The model under review builds one solid part; all positions refer to its coordinate system, in mm. Face numbers are marked on the shaded views. Coordinates: 2 decimals unless noted, no trailing zeros. Loops run counter-clockwise (first coordinate to the right, second up) from the corner with the lowest first, then second, coordinate; pieces in that order, holes last. Notation, with made-up numbers: M 86.25,55.25 L 106.25,55.25 A16 ccw 106.25,65.25 Z; hole C 12,41 d6. An arc over 180 degrees is marked long. Use one line per item in the form item = value.
Autodesk Inventor part; units mm, degrees
ref_plane "作業平面1" through (0, -0.65, 0) normal (0, 1, 0) x (1, 0, 0)
ref_plane "YZ Plane" through (0, 0, 0) normal (1, 0, 0) x (0, 1, 0)
ref_plane "XZ Plane" through (0, 0, 0) normal (0, 1, 0) x (-1, 0, 0)
sketch "スケッチ1" plane through (0, 0, 0) normal (0, 1, 0) x (-1, 0, 0)
  circle A0 centre (0, 0) radius 8.9
  line L0 (0, -8.9) -> (63.2748, -8.9)
  line L1 (63.2748, -8.9) -> (63.2748, 8.9)
  line L2 (63.2748, 8.9) -> (0, 8.9)
  line L3 (0, 8.9) -> (0, -8.9)
  circle A1 centre (0, 0) radius 8.4
  line L4 (0, -8.4) -> (63.2748, -8.4)
  line L5 (63.2748, -8.4) -> (63.2748, 8.4)
  line L6 (63.2748, 8.4) -> (0, 8.4)
  line L7 (0, 8.4) -> (0, -8.4)
  point P0 (0, 8.4)
  point P1 (0, 8.9)
  dimension "d0" = 17.8
  dimension "d1" = 16.8
extrude "押し出し1" add sketch "スケッチ1" along normal blind 0.85 contours L3 A1 A0 | L2 L1 L6 A0 | A0 L6 L3 | L3 L4 A0 | A0 L4 L1 L0
sketch "スケッチ2" plane through (0, 0.85, 0) normal (0, 1, 0) x (1, 0, 0)
  circle A0 centre (0, 0) radius 12
  line L0 (0, 12) -> (-63.2748, 12)
  line L1 (-63.2748, 12) -> (-63.2748, -12)
  line L2 (-63.2748, -12) -> (0, -12)
  line L3 (0, -12) -> (0, 12)
  line L4 (-63.2748, 8.9) -> (-63.2748, 8.4)
  line L5 (-63.2748, 8.4) -> (0, 8.4)
  line L6 (0, -8.4) -> (-63.2748, -8.4)
  arc A1 (0, -8.4) -> (0, 8.4) centre (0, 0) ccw
  point P0 (0, -12)
  dimension "d4" = 24
extrude "押し出し2" add sketch "スケッチ2" along normal blind 1 contours A0 L3 A1 | L3 L5 A0 | A0 L5 L1 L0 | L2 L1 L6 A0 | A0 L6 L3
mirror "ミラー1" about plane through (-27.1874, 0, 0) normal (0, -1, 0)
sketch "スケッチ3" plane through (0, 1.85, 0) normal (0, 1, 0) x (1, 0, 0)
  line L0 (-14.7409, 17.0236) -> (-35.8476, -19.5343)
  line L1 (0, -8.4) -> (-63.2748, -8.4)
  line L2 (-63.2748, -8.4) -> (-63.2748, -12)
  line L3 (-63.2748, -12) -> (0, -12)
  arc A0 (0, -12) -> (0, 12) centre (0, 0) ccw
  line L4 (0, 12) -> (-63.2748, 12)
  line L5 (-63.2748, 12) -> (-63.2748, 8.4)
  line L6 (-63.2748, 8.4) -> (0, 8.4)
  arc A1 (0, -8.4) -> (0, 8.4) centre (0, 0) ccw
  point P0 (-31.4977, -12)
  point P1 (-29.4192, -8.4)
  point P2 (-19.7197, 8.4)
  point P3 (-17.6412, 12)
extrude "押し出し3" cut sketch "スケッチ3" against normal through all contours L0 L6 L5 L4 | L0 L3 L2 L1
ref_plane "作業平面1" through (0, -0.65, 0) normal (0, 1, 0) x (1, 0, 0)
sketch "スケッチ4" plane through (0, -0.65, 0) normal (0, 1, 0) x (1, 0, 0)
  line L0 (-19.7197, 8.4) -> (0, 8.4)
  arc A0 (0, -8.4) -> (0, 8.4) centre (0, 0) ccw
  line L1 (0, -8.4) -> (-29.4192, -8.4)
  line L2 (-19.7197, 8.4) -> (-29.4192, -8.4)
  circle A1 centre (0, 0) radius 1.6
  dimension "d10" = 3.2
extrude "押し出し4" add sketch "スケッチ4" along normal up to surface (2.5 mm away)
fillet "フィレット1" radius 1 3 edges at (-9.8599, -0.65, -8.4) (8.4, -0.65, 0) (-14.7096, -0.65, 8.4)
sketch "スケッチ5" plane through (0, 1.85, 0) normal (0, 1, 0) x (1, 0, 0)
  circle A0 centre (-27.8315, -17.35) radius 1.6
  circle A1 centre (-8.7282, 17.4379) radius 1.6
  line L0 (0, 12) -> (-17.6412, 12)
  line L1 (-17.6412, 12) -> (-10.5885, 24.2158)
  line L2 (-10.5885, 24.2158) -> (0, 24.2158)
  line L3 (-39.933, -26.6105) -> (-10.6554, 24.0998)
  line L4 (0, 12) -> (-17.6412, 12)
  circle A2 centre (0, 0) radius 24.2158
  arc A3 (0, -12) -> (0, 12) centre (0, 0) ccw
  line L5 (11.4695, 3.5285) -> (5.2849, 23.6321)
  circle A4 centre (1.9592, 17.4379) radius 1.6
  line L6 (-39.933, -26.6105) -> (-10.6554, 24.0998)
  circle A5 centre (-31.9338, -24.4553) radius 1.6
  circle A6 centre (-36, -34.6362) radius 1.6
  circle A7 centre (-27.8315, -17.35) radius 1.6
  line L7 (-39.933, -26.6105) -> (-10.6554, 24.0998)
  line L8 (-40, -50) -> (-40, -26.8605)
  line L9 (-38, -50.5) -> (-39.5, -50.5)
  line L10 (-31, -42) -> (-31, -32.0566)
  line L11 (-30.933, -31.8066) -> (-18.1986, -9.75)
  line L12 (-37.5, -50) -> (-37.5, -43)
  line L13 (-37, -42.5) -> (-31.5, -42.5)
  circle A8 centre (-31.9338, -24.4553) radius 5.85
  arc A9 (19.2639, -16.134) -> (19.9469, -15.951) centre (19.5139, -15.701) ccw
  line L14 (29.8557, 1.2115) -> (19.9469, -15.951)
  arc A10 (29.8557, 1.2115) -> (29.8557, 1.7115) centre (29.4226, 1.4615) ccw
  line L15 (10.25, 35.6695) -> (29.8557, 1.7115)
  arc A11 (10.25, 35.6695) -> (9.567, 35.8525) centre (9.817, 35.4195) ccw
  line L16 (-10.4724, 24.2828) -> (9.567, 35.8525)
  arc A12 (-10.4724, 24.2828) -> (-10.6554, 24.0998) centre (-10.2224, 23.8498) ccw
  arc A13 (-39.933, -26.6105) -> (-40, -26.8605) centre (-39.5, -26.8605) ccw
  arc A14 (-40, -50) -> (-39.5, -50.5) centre (-39.5, -50) ccw
  arc A15 (-38, -50.5) -> (-37.5, -50) centre (-38, -50) ccw
  arc A16 (-37, -42.5) -> (-37.5, -43) centre (-37, -43) ccw
  arc A17 (-31.5, -42.5) -> (-31, -42) centre (-31.5, -42) ccw
  arc A18 (-30.933, -31.8066) -> (-31, -32.0566) centre (-30.5, -32.0566) ccw
  arc A19 (-17.7656, -9.5) -> (-18.1986, -9.75) centre (-17.7656, -10) ccw
  line L17 (-17.7656, -9.5) -> (7.6395, -9.5)
  arc A20 (7.8895, -9.567) -> (7.6395, -9.5) centre (7.6395, -10) ccw
  line L18 (7.8895, -9.567) -> (19.2639, -16.134)
  circle A21 centre (1.9592, 17.4379) radius 1.6
  circle A22 centre (24.5152, 1.2615) radius 1.6
  circle A23 centre (5.1388, 27.5224) radius 1.6
  circle A24 centre (13.1994, 17.561) radius 1.6
  circle A25 centre (20.4199, -5.8317) radius 1.6
  circle A26 centre (-8.7282, 17.4379) radius 1.6
  circle A27 centre (0, 0) radius 1.5
  point P0 (0, 24.2158)
  point P1 (-20.2427, -13.2905)
  point P2 (-12.6465, 20.6512)
  point P3 (-37, -21.5303)
  point P4 (-29.8432, -29.9191)
  point P5 (-26.1568, -23.5339)
  dimension "d14" = 15
  dimension "d15" = 3.2
  dimension "d16" = 5
extrude "押し出し5" add sketch "スケッチ5" against normal blind 1 contours A1 | A3 L17 A19 L11 A2 L3 L0 | L0 L1 A2 L5 A3 | L5 A2 A22 L18 A20 L17 A3 | L1 A12 L2 A2 | A2 L11 A8 L3 | A2 L2 A12 L16 A11 L15 A10 L14 A9 L18 A22 | L1 L2 A12 | A8 L11 A18 L10 A17 L13 A16 L12 A15 L9 A14 L8 A13 L3 | A8 L11 | A22 A2 | A2 A22 | A8 L11 | A4 | A6 | A23 | A24 | A25 | A27
sketch "スケッチ6" plane through (0, 1.85, 0) normal (0, 1, 0) x (1, 0, 0)
  line L0 (-19.4977, -12) -> (0, -12)
  line L1 (-19.4977, -12) -> (-17.7656, -9)
  line L2 (-17.7656, -9) -> (7.9373, -9)
  arc A0 (0, -12) -> (0, 12) centre (0, 0) ccw
  line L3 (-29.8432, -29.9191) -> (-19.4977, -12)
  point P0 (-25.741, -22.8137)
  point P1 (-20.2427, -13.2905)
  point P2 (-31, -31.9226)
  dimension "d19" = 3
extrude "押し出し6" cut sketch "スケッチ6" against normal through all
sketch "スケッチ7" plane through (0, -1.85, 0) normal (0, -1, 0) x (1, 0, 0)
  line L0 (-19.3733, -9) -> (0, -9)
  line L1 (-17.7656, 9) -> (-19.4977, 12)
  line L2 (-31.4977, 12) -> (-19.4977, 12)
  line L3 (-31.4977, 12) -> (-29.4192, 8.4)
  line L4 (0, 8.4) -> (-29.4192, 8.4)
  arc A0 (0, -8.4) -> (0, 8.4) centre (0, 0) ccw
  line L5 (-19.7197, -8.4) -> (0, -8.4)
  line L6 (-19.7197, -8.4) -> (-17.6412, -12)
  line L7 (0, -12) -> (-17.6412, -12)
  arc A1 (0, -12) -> (7.9373, 9) centre (0, 0) ccw
  line L8 (7.9373, 9) -> (-17.7656, 9)
  circle A2 centre (0, 0) radius 1.6
  line L9 (0, -7.4) -> (-20.2971, -7.4)
  arc A3 (0, -7.4) -> (0, 7.4) centre (0, 0) ccw
  line L10 (-28.8418, 7.4) -> (0, 7.4)
  line L11 (-20.2971, -7.4) -> (-28.8418, 7.4)
  circle A4 centre (0, 0) radius 9
  line L12 (-17.7656, 9) -> (7.9373, 9)
  line L13 (-10.5631, -24.2158) -> (-10.5885, -24.2158)
  arc A5 (-26.1568, 23.5339) -> (-29.8432, 29.9191) centre (-31.9338, 24.4553) ccw
  line L14 (-26.1568, 23.5339) -> (-17.7656, 9)
  circle A6 centre (-27.8315, 17.35) radius 1.6
  circle A7 centre (-31.9338, 24.4553) radius 1.6
  arc A8 (7.9373, 9) -> (7.3314, 9.5) centre (0, 0) ccw
  line L15 (7.3314, 9.5) -> (7.6395, 9.5)
  arc A9 (7.6395, 9.5) -> (7.8895, 9.567) centre (7.6395, 10) ccw
  line L16 (7.8895, 9.567) -> (19.2639, 16.134)
  arc A10 (19.9469, 15.951) -> (19.2639, 16.134) centre (19.5139, 15.701) ccw
  line L17 (19.9469, 15.951) -> (29.8557, -1.2115)
  arc A11 (29.8557, -1.7115) -> (29.8557, -1.2115) centre (29.4226, -1.4615) ccw
  line L18 (29.8557, -1.7115) -> (10.25, -35.6695)
  arc A12 (9.567, -35.8525) -> (10.25, -35.6695) centre (9.817, -35.4195) ccw
  line L19 (9.567, -35.8525) -> (-10.4724, -24.2828)
  arc A13 (-10.5631, -24.2158) -> (-10.4724, -24.2828) centre (-10.2224, -23.8498) ccw
  line L20 (-10.5885, -24.2158) -> (-39.933, 26.6105)
  arc A14 (-40, 26.8605) -> (-39.933, 26.6105) centre (-39.5, 26.8605) ccw
  line L21 (-40, 26.8605) -> (-40, 50)
  arc A15 (-39.5, 50.5) -> (-40, 50) centre (-39.5, 50) ccw
  line L22 (-39.5, 50.5) -> (-38, 50.5)
  arc A16 (-37.5, 50) -> (-38, 50.5) centre (-38, 50) ccw
  line L23 (-37.5, 50) -> (-37.5, 43)
  arc A17 (-37.5, 43) -> (-37, 42.5) centre (-37, 43) ccw
  line L24 (-37, 42.5) -> (-31.5, 42.5)
  arc A18 (-31, 42) -> (-31.5, 42.5) centre (-31.5, 42) ccw
  line L25 (-31, 42) -> (-31, 32.0566)
  arc A19 (-31, 32.0566) -> (-30.933, 31.8066) centre (-30.5, 32.0566) ccw
  line L26 (-30.933, 31.8066) -> (-29.8432, 29.9191)
extrude "押し出し7" cut sketch "スケッチ7" against normal up to surface (2.7 mm away) contours L6 L5 A4 L0 | L0 A4 L8 A1 L7 L6 | A4 L5 A0 L4 | L11 L10 A4 L9 | A4 L4 L3 L2 L1 L8 | A4 L10 A3 L9 | A2
properties part number "screw_cover_upper"
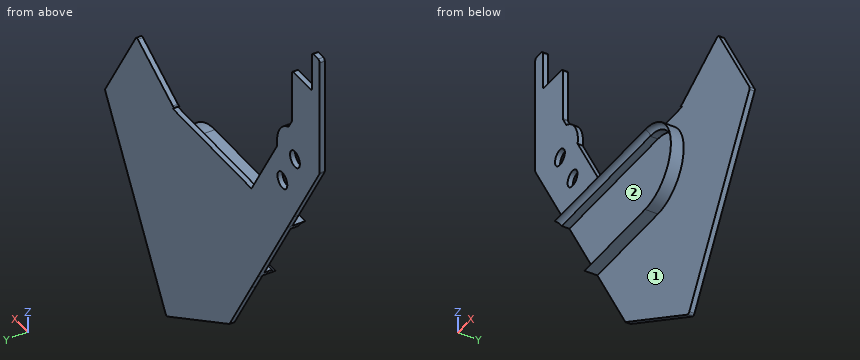
1. Add section B-B (z = 0). State the section outline as (x, y) points, then the cut area to 3 significant figures.
Response values:
outline = M -24.57,0.85 L 7.4,0.85 L 7.4,-0.65 A1 cw 8.4,-1.65 L 8.4,0.85 L 29.16,0.85 L 29.16,1.85 L -24.57,1.85 Z
area = 55.4 mm^2
2. Add section C-C (x = 16.5). State the section outline as (y, z) points.
Response values:
outline = M 0.85,-24.84 L 1.85,-24.84 L 1.85,14.54 L 0.85,14.54 Z
3. Insertion check: P1, Ø2, axis at x = 2, y = 1.5, coming from the -Z side; P2, Ø2, axis at x = -14, y = -0.5, coming from the -Z side; P3, Ø5, axis at x = -27.83, z = 17.35, coming from the +Y side; P4, Ø0.8, axis at x = -34.5, y = 1, coming from the +Z side. Each pin has a flat end and moves straight along its axis. Give the tip position at first contact, or say it passes through.
Response values:
P1 = -32.06
P2 = -8.4
P3 = 1.85
P4 = 42.5
4. Add section D-D (z = 45.5). State the section outline as (x, y) points, then the cut area to 3 significant figures.
Response values:
outline = M -40,0.85 L -37.5,0.85 L -37.5,1.85 L -40,1.85 Z
area = 2.50 mm^2
5. The part is to be moulded in two halves that separate along Z. For the marked faces 1 and 2, say which applies: pulls with the +Z half, pulls with the -Z half, needs draft (parallel to the pull), parting line crosses it, or undercut.
Response values:
face_1 = needs draft
face_2 = undercut
6. Add section A-A (z = 17.35). State the section outline as (x, y) points.
Response values:
outline = M -34.59,0.85 L -29.43,0.85 L -29.43,1.85 L -34.59,1.85 Z; M -26.23,0.85 L -22.59,0.85 L -22.59,1.85 L -26.23,1.85 Z
7. Wall thickness on line 1 along Z through (x, y) = (-1, 0.6); line 2 along X through (y, z) = (1.3, 44); line 3 along Y through (x, z) = (-6, -7.5): over which ranges is each line inside the solid? List them lowest first. Write a range as from..to.
Response values:
line_1 = -8.4..-7.4, 7.4..8.4
line_2 = -40..-37.5
line_3 = -0.66..1.85
